```python
from build123d import *

# Parameters (mm, degrees)
F0_R           = 7.6
F1_DEPTH       = 5
F2_R           = 7.6
F3_DEPTH       = 60
F4_R           = 5
F6_D           = 3.5
F6_CSINK_D     = 8
F6_CSINK_ANGLE = 90
F7_R           = 2


with BuildPart() as f1:
    # F0 (on Top) → F1 (new body)
    with BuildSketch(Plane.XY):
        with BuildLine():
            Line((30, -7.691861), (7.293509, -7.691861))
            ThreePointArc((7.293509, -7.691861), (0, 10.6), (-7.293509, -7.691861))
            Line((-7.293509, -7.691861), (-30, -7.691861))
            Line((-30, -7.691861), (-30, -10.6))
            Line((-30, -10.6), (0, -10.6))
            Line((0, -10.6), (30, -10.6))
            Line((30, -10.6), (30, -7.691861))
        make_face()
        Circle(F0_R, mode=Mode.SUBTRACT)
        Circle(F0_R)
    extrude(amount=F1_DEPTH)

    # F2 (on face) → F3 (join)
    with BuildSketch(Plane.XY.offset(5)):
        with BuildLine():
            Line((30, -7.691861), (7.293509, -7.691861))
            ThreePointArc((7.293509, -7.691861), (0, 10.6), (-7.293509, -7.691861))
            Line((-7.293509, -7.691861), (-30, -7.691861))
            Line((-30, -7.691861), (-30, -10.6))
            Line((-30, -10.6), (30, -10.6))
            Line((30, -10.6), (30, -7.691861))
        make_face()
        Circle(F2_R, mode=Mode.SUBTRACT)
    extrude(amount=F3_DEPTH)

    # F4
    f4_edges = [f1.edges().sort_by_distance(p)[0] for p in [
        (-7.293509, -7.691861, 32.5),
        (7.293509, -7.691861, 32.5),
    ]]
    fillet(f4_edges, radius=F4_R)

    # F6 (through all)
    with Locations(Plane(origin=(0, -7.691861, 0), x_dir=(-1, 0, 0), z_dir=(0, 1, 0))):
        with Locations((-22.682999, 50), (-22.682999, 15), (22.682999, 50), (22.682999, 15)):
            CounterSinkHole(F6_D / 2, F6_CSINK_D / 2, counter_sink_angle=F6_CSINK_ANGLE)

    # F7
    f7_edges = [f1.edges().sort_by_distance(p)[0] for p in [
        (0, 10.6, 65),
        (-30, -7.691861, 32.5),
        (30, -7.691861, 32.5),
        (22.682999, -7.691861, 0),
        (0, 10.6, 0),
    ]]
    fillet(f7_edges, radius=F7_R)


solid = f1.part
```
Input: part model. Units: mm. Frame: model coordinates. A direction names the side the tool comes from. Coordinates: 2 decimals unless noted, no trailing zeros. Order: outer loops, then holes, each group sorted by start corner. A loop starts at its lowest first (then second) coordinate and runs counter-clockwise, first axis right, second up. Notation, with made-up numbers: (-27.5, -39) - (-3.5, -39) arc R14 ccw to (-3.5, -20) - close; hole circle Ø5 at (39, 54.5). An arc over 180 degrees is marked (long way). Put each result on its own line as item: value.
1. Cut plane A-A on z = 50. Return the cut outline in (x, y), then the cut area to 3 significant figures.
Report:
outline: (-30, -10.6) - (-24.43, -10.6) - (-24.43, -9.94) - (-26.68, -7.69) - (-28, -7.69) arc R2 ccw to (-30, -9.69) - close; (-20.93, -10.6) - (20.93, -10.6) - (20.93, -9.94) - (18.68, -7.69) - (15.37, -7.69) arc R5 cw to (10.44, -1.83) arc R10.6 ccw (long way) to (-10.44, -1.83) arc R5 cw to (-15.37, -7.69) - (-18.68, -7.69) - (-20.93, -9.94) - close; (24.43, -10.6) - (30, -10.6) - (30, -9.69) arc R2 ccw to (28, -7.69) - (26.68, -7.69) - (24.43, -9.94) - close; hole circle Ø15.2 at (0, 0)
area: 308 mm2
2. Line query: line 1 along X through (y, z) = (-10.15, 50); line 2 along Z through (x, y) = (22.5, -9); line 3 along Y through (x, z) = (-27, 25). Output: solid intervals per line, ascending.
Report:
line 1: x = -30 to -24.43, -20.93 to 20.93, 24.43 to 30
line 2: z = 0.12 to 12.31, 17.69 to 47.31, 52.69 to 64.88
line 3: y = -10.6 to -7.69
3. Draft query along X for faces 5 (the face through (22, -7.692, 32)), 6 (the face through (29.399, -8.262, 32.045)), 7 (the face through (-24.54, -9.833, 15.082)), 8 (the face through (-21.742, -10.276, 16.476)). Return one class per face: pulls with the +X half, pulls with the -X half, needs draft (parallel to the pull), parting line crosses it, or undercut.
Report:
face 5: needs draft
face 6: pulls with the +X half
face 7: undercut
face 8: undercut
4. Cut plane D-D on y = -8.5. State how many separate pieces and enclosed holes the cut face has, then the cut area to 3 significant figures.
Report:
separate pieces: 1
enclosed holes: 4
area: 3,700 mm2
5. Cut plane B-B on x = 0. Return the cut outline in (y, z).
Report:
outline: (-10.6, 0) - (8.6, 0) arc R2 ccw to (10.6, 2) - (10.6, 63) arc R2 ccw to (8.6, 65) - (7.6, 65) - (7.6, 5) - (-7.6, 5) - (-7.6, 65) - (-10.6, 65) - close
6. Reachability of faces 1 (the face through (22.581, -8.262, 64.399)), 2 (the face through (-22.785, -8.262, 64.399)), 3 (the face through (-22, -7.692, 32)), 4 (the face through (-22.785, -8.262, 0.601)) from +Z, -Z, +X, -X, +Y, -Y: full face, straight path, thin tool, end or side. Return the list, or none.
Report:
face 1: +Z, +X, +Y
face 2: +Z, -X, +Y
face 3: +Z, -Z, -X, +Y
face 4: -Z, -X, +Y
7. Cut plane C-C on z = 7.5. Return the cut outline in (x, y), then the cut area to 3 significant figures.
Report:
outline: (-30, -10.6) - (30, -10.6) - (30, -9.69) arc R2 ccw to (28, -7.69) - (15.37, -7.69) arc R5 cw to (10.44, -1.83) arc R10.6 ccw (long way) to (-10.44, -1.83) arc R5 cw to (-15.37, -7.69) - (-28, -7.69) arc R2 ccw to (-30, -9.69) - close; hole circle Ø15.2 at (0, 0)
area: 339 mm2
8. Contact query for flat-ended pins moving along their axis: pin 1 Ø4 at (x, z) = (-22.68, 15) entering from +Y; pin 2 Ø6 at (y, z) = (-3, 23.5) entering from -X; pin 3 Ø1.5 at (x, z) = (14.5, 45.5) entering from +Y; pin 4 Ø3 at (x, z) = (22.68, 50) entering from -Y. Output: stop coordinate, or through.
Report:
pin 1: stops at y = -9.69
pin 2: stops at x = -11.62
pin 3: stops at y = -7.42
pin 4: passes through
